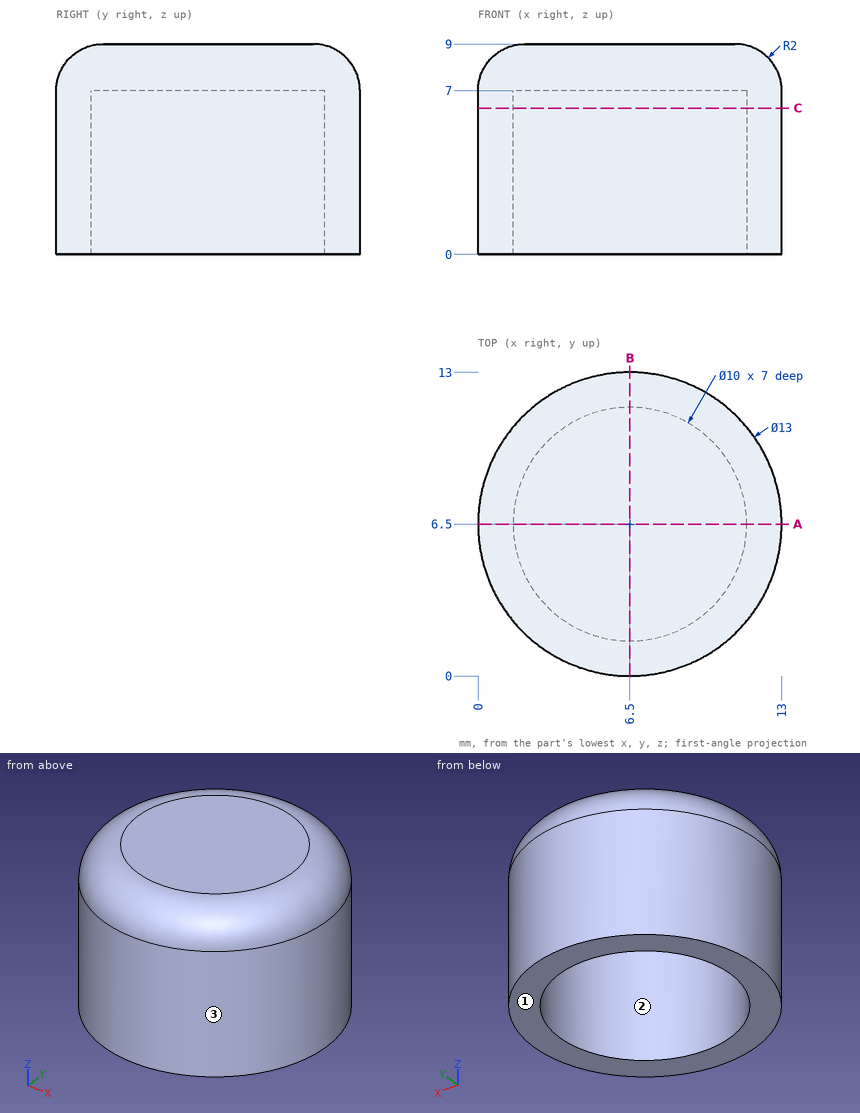
Design review of the part shown in the three views and the two pictorial views. Dimensions are in mm from the part's minimum x, y and z. Coordinates: 2 decimals unless noted, no trailing zeros. Write each loop counter-clockwise with the first axis right and the second up, starting at its lowest first coordinate (ties: lowest second). Pieces come first, ordered by that corner, then holes. Notation, with made-up numbers: (78.5, 44.25) -> (121.5, 44.25) arc R15 cw to (121.5, 61.25) -> close; hole circle Ø1 at (-6.5, -22). An arc over 180 degrees is marked (long way). Answer in a Markdown table with one row per item.
1. We need section C-C, the plane z = 6.25. State the section outline as (x, y) points.
Answers below:
| item | result |
|---|---|
| outline | circle Ø13 at (6.5, 6.5); hole circle Ø10 at (6.5, 6.5) |
2. Clearance check with a flat-ended pin moving along its axis: pin 1 Ø1 at (x, y) = (7.5, 5) entering from -Z. State where the tip first meets the part, or that it passes through.
Answers below:
| item | result |
|---|---|
| pin 1 | stops at z = 7 |
3. Draft analysis for pull direction X (two halves, no side actions). For the marked faces 1, 2 and 3, state which applies: +X half, -X half, draft (parallel to the pull), parting line (faces both ways), or undercut.
Answers below:
| item | result |
|---|---|
| face 1 | draft |
| face 2 | undercut |
| face 3 | parting line |
4. Wall thickness on probe 1 along Y at (x, z) = (6.5, 2.5); probe 2 along X at (y, z) = (7.5, 2); probe 3 along Y at (x, z) = (5.75, 6.25): over which ranges is each line inside the solid? List them lowest first. Write a range as [from, to].
Answers below:
| item | result |
|---|---|
| probe 1 | y = [0, 1.5], [11.5, 13] |
| probe 2 | x = [0.08, 1.6], [11.4, 12.92] |
| probe 3 | y = [0.04, 1.56], [11.44, 12.96] |
5. We need section A-A, the plane y = 6.5. State the section outline as (x, z) points, and give its area (3 significant figures).
Answers below:
| item | result |
|---|---|
| outline | (0, 0) -> (1.5, 0) -> (1.5, 7) -> (11.5, 7) -> (11.5, 0) -> (13, 0) -> (13, 7) arc R2 ccw to (11, 9) -> (2, 9) arc R2 ccw to (0, 7) -> close |
| area | 45.3 mm^2 |
